from build123d import *

# Parameters (mm, degrees)
SKETCH4_R   = 2.794
SKETCH4_R_2 = 2.54


with BuildPart() as part:
    # Sweep-Thin1: sweep along a path in Sketch2
    with BuildLine(Plane(origin=(0, 0, 0), x_dir=(1, 0, 0), z_dir=(0, 1, 0))) as sweep_thin1_path:
        Line((0, 0), (0, 152.4))
        ThreePointArc((0, 152.4), (7.439487758, 170.360512242), (25.4, 177.8))
        Line((25.4, 177.8), (50.8, 177.8))
    # Sketch4 → Sweep-Thin1 (sweep)
    with BuildSketch(Plane.XY):
        Circle(SKETCH4_R)
        Circle(SKETCH4_R_2, mode=Mode.SUBTRACT)
    sweep(path=sweep_thin1_path.line)


solid = part.part
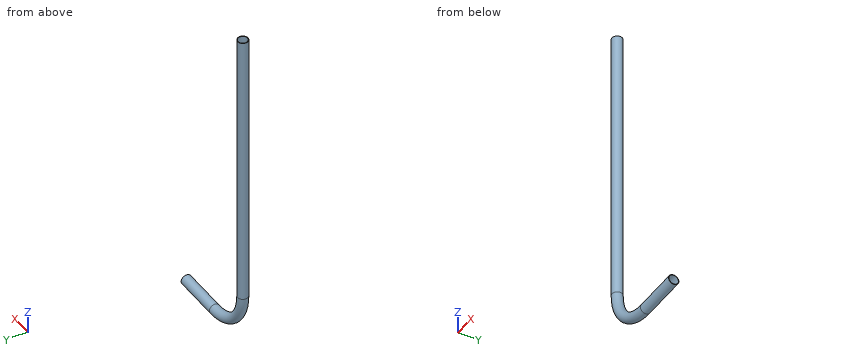
Input: part model. Units: mm. Frame: model coordinates. Give positions to 0.01 mm unless a question says otherwise; leave off trailing zeros. Order: outer loops, then holes, each group sorted by start corner. A loop starts at its lowest first (then second) coordinate and runs counter-clockwise, first axis right, second up. Notation, with made-up numbers: (19.5, 79) - (38.5, 79) arc R14 cw to (38.5, 101) - close; hole circle Ø7 at (3.5, 83.25). An arc over 180 degrees is marked (long way). Write each question's results on one line, items separated by ' | '.
Item 1: Contact query for flat-ended pins moving along their axis: pin 1 Ø1.5 at (y, z) = (-1.5, -155.5) entering from -X; pin 2 Ø1 at (y, z) = (1.5, -80.5) entering from -X; pin 3 Ø2 at (x, y) = (11, -2) entering from -Z. Output: stop coordinate, or through.
A:
pin 1: stops at x = -2.53 | pin 2: stops at x = -2.61 | pin 3: stops at z = -176.68
Item 2: Material intervals for line 1 along Y through (x, z) = (38, -177.8); line 2 along Z through (x, y) = (36.5, 0), sorted ascending.
A:
line 1: y = -2.79 to -2.54, 2.54 to 2.79 | line 2: z = -180.59 to -180.34, -175.26 to -175.01
Item 3: Section A-A (y = 0). Return loops of the section in (x, z).
A:
outline: (-2.79, -152.4) arc R28.19 ccw to (25.4, -180.59) - (50.8, -180.59) - (50.8, -180.34) - (25.4, -180.34) arc R27.94 cw to (-2.54, -152.4) - (-2.54, 0) - (-2.79, 0) - close; (2.54, -152.4) arc R22.86 ccw to (25.4, -175.26) - (50.8, -175.26) - (50.8, -175.01) - (25.4, -175.01) arc R22.61 cw to (2.79, -152.4) - (2.79, 0) - (2.54, 0) - close
Item 4: Section B-B (z = -21.5). Return loops of the section in (x, y).
A:
outline: circle Ø5.59 at (0, 0); hole circle Ø5.08 at (0, 0)
Item 5: Section C-C (x = 34). Return loops of the section in (y, z).
A:
outline: circle Ø5.59 at (0, -177.8); hole circle Ø5.08 at (0, -177.8)
